Read the model definition and answer for the solid it produces. Units are mm, in the model's axes. Face numbers are marked on the shaded views. A direction names the side the tool comes from. Coordinates: 2 decimals unless noted, no trailing zeros. Write each loop counter-clockwise with the first axis right and the second up, starting at its lowest first coordinate (ties: lowest second). Pieces come first, ordered by that corner, then holes. Notation, with made-up numbers: (21.25, 87) - (68.25, 87) arc R13 cw to (68.25, 96) - close; hole circle Ø5 at (12, 9). An arc over 180 degrees is marked (long way). Return JSON: item names as keys, results as strings.
```python
from build123d import *

# Parameters (mm, degrees)
F1_DEPTH = 36.83
F2_R     = 5.08
F3_R     = 5.08


with BuildPart() as f1:
    # F0 (on Front) → F1 (new body)
    with BuildSketch(Plane.XZ):
        Polygon((-20.186856, 15.762338), (-42.862501, 15.762338), (-42.862501, -20.186855), (51.158469, -20.186855), (51.158469, 15.762338), (25.901856, 15.762338), (25.901856, 40.097181), (-20.186856, 40.097181), align=None)
    extrude(amount=F1_DEPTH)

    # F2
    f2_edges = [f1.edges().sort_by_distance(p)[0] for p in [
        (25.901856, -18.415, 40.097181),
        (-20.186856, -18.415, 40.097181),
        (51.158469, -18.415, 15.762338),
        (25.901856, -18.415, 15.762338),
        (-20.186856, -18.415, 15.762338),
        (-42.862501, -18.415, 15.762338),
    ]]
    fillet(f2_edges, radius=F2_R)

    # F3
    f3_edges = [f1.edges().sort_by_distance(p)[0] for p in [
        (-31.524679, -36.83, 15.762338),
        (-21.674754, -36.83, 17.250236),
        (-41.374603, -36.83, 14.274441),
        (-20.186856, -36.83, 27.92976),
        (-42.862501, -36.83, -4.752258),
        (-18.698959, -36.83, 38.609283),
        (4.147984, -36.83, -20.186855),
        (2.8575, -36.83, 40.097181),
        (51.158469, -36.83, -4.752258),
        (24.413958, -36.83, 38.609283),
        (49.670572, -36.83, 14.274441),
        (25.901856, -36.83, 27.92976),
        (38.530163, -36.83, 15.762338),
        (27.389753, -36.83, 17.250236),
    ]]
    fillet(f3_edges, radius=F3_R)


solid = f1.part
```
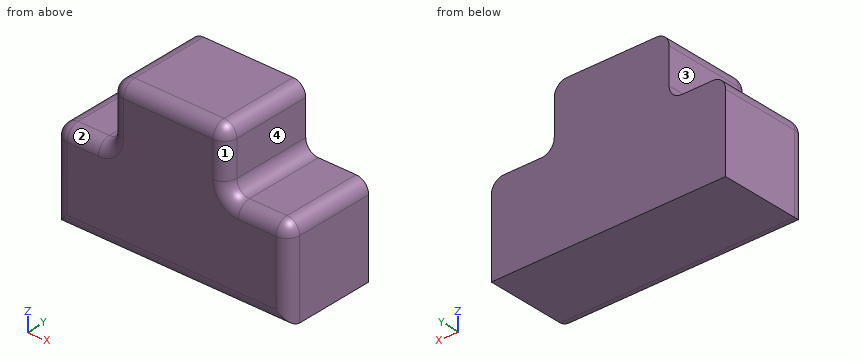
(1) A cutting plane is placed at B-B (x = 41). Determine the outline of the cut face in (y, z), and give its area (3 significant figures).
Answer:
{"outline": "(-36.83, -15.11) arc R5.08 ccw to (-31.75, -20.19) - (0, -20.19) - (0, 15.76) - (-31.75, 15.76) arc R5.08 ccw to (-36.83, 10.68) - close", "area": "1,310 mm²"}
(2) A cutting plane is placed at C-C (z = 22.5). Determine the outline of the cut face in (x, y), and give its area (3 significant figures).
Answer:
{"outline": "(-20.19, -31.75) arc R5.08 ccw to (-15.11, -36.83) - (20.82, -36.83) arc R5.08 ccw to (25.9, -31.75) - (25.9, 0) - (-20.19, 0) - close", "area": "1,690 mm²"}
(3) Flat-ended cylindrical pins translate along their axes: P1, Ø7.5, axis at x = 36.5, y = -10.5, coming from the +Z side; P2, Ø1.5, axis at x = -19, y = -18, coming from the +Z side; P3, Ø4.5, axis at y = -17, z = 29, coming from the -X side; P4, Ø3, axis at x = 30.5, z = 10.5, coming from the +Y side. Find the tip coordinate at first contact, or state that the pin passes through.
Answer:
{"P1": "z = 15.76", "P2": "z = 39.01", "P3": "x = -20.19", "P4": "y = 0"}
(4) Which of the six approach directions +Z, -Z, +X, -X, +Y, -Y give full straight-line access (tool end or side, diameter ignored) to the marked faces 1, 2, 3 and 4?
Answer:
{"face 1": "+Z, +X, -Y", "face 2": "+Z, -X, -Y", "face 3": "+Z, -X, +Y, -Y", "face 4": "+Z, +X, +Y, -Y"}
(5) A cutting plane is placed at A-A (y = -24.5). Determine the outline of the cut face in (x, z), and give its area (3 significant figures).
Answer:
{"outline": "(-42.86, -20.19) - (51.16, -20.19) - (51.16, 10.68) arc R5.08 ccw to (46.08, 15.76) - (30.98, 15.76) arc R5.08 cw to (25.9, 20.84) - (25.9, 35.02) arc R5.08 ccw to (20.82, 40.1) - (-15.11, 40.1) arc R5.08 ccw to (-20.19, 35.02) - (-20.19, 20.84) arc R5.08 cw to (-25.27, 15.76) - (-37.78, 15.76) arc R5.08 ccw to (-42.86, 10.68) - close", "area": "4,490 mm²"}
(6) Straight lines are drawn through the part: line 1 (X direction, y = -11, z = 27.5); line 2 (Z direction, x = -31.5, y = -9); line 3 (Z direction, x = 31, y = -35). For each, find the intervals that lie inside material, in ascending order. Write a range as from..to.
Answer:
{"line 1": "-20.19..25.9", "line 2": "-20.19..15.76", "line 3": "-19.01..14.59"}
